Read the model definition and answer for the solid it produces. Units are mm, in the model's axes. Coordinates: 2 decimals unless noted, no trailing zeros. Write each loop counter-clockwise with the first axis right and the second up, starting at its lowest first coordinate (ties: lowest second). Pieces come first, ordered by that corner, then holes. Notation, with made-up numbers: (43.25, -24) -> (72.25, -24) arc R18 ccw to (72.25, -12) -> close; hole circle Ø10 at (-21.5, -27.75). An arc over 180 degrees is marked (long way). Write item = value, one per line. Start each with the question number.
1) Section B-B (x = 51) is taken. Determine the outline of the cut face in (y, z) (3 decimals).
2) For a pull along Y with two mould halves and no side action, classify faces 1 (the face through (6, -34, 0)), 2 (the face through (-6, -32.3, 0.5)) as released by +Y, released by -Y, zero draft, split by the parting line, or undercut.
3) Section C-C (z = 0.75) is taken. Determine the outline of the cut face in (x, y).
4) Section A-A (y = -4.5) is taken. Determine the outline of the cut face in (x, z).
5) A flat-ended cylindrical pin translates along its axis: pin 1 Ø6 at (x, y) = (-39, 26.5) entering from +Z. Find the tip coordinate at first contact, or state that the pin passes through.
6) Find the intervals of material crossed by line 1 along X through (y, z) = (7, 0.35); line 2 along Y through (x, z) = (65.5, 0.2) (3 decimals); line 3 along X through (y, z) = (-11, 0.9), in increasing order. Write a range as from..to.
from build123d import *

# Parameters (mm, degrees)
F0_W     = 152
F0_H     = 73
F1_DEPTH = 1
F0_W_2   = 150
F0_H_2   = 64.29
F2_DEPTH = 0.5


with BuildPart() as f1:
    # F0 (on Top) → F1 (new body)
    with BuildSketch(Plane.XY):
        Polygon((-78, -30), (-78, -38), (78, -38), (78, -30), (81, -30), (81, 38), (-81, 38), (-81, -30), align=None)
        Rectangle(F0_W, F0_H, mode=Mode.SUBTRACT)
    extrude(amount=F1_DEPTH)

    # F0 (on Top) → F2 (join)
    with BuildSketch(Plane.XY):
        Rectangle(F0_W, F0_H)
        Rectangle(F0_W_2, F0_H_2, mode=Mode.SUBTRACT)
    extrude(amount=F2_DEPTH)


solid = f1.part
Answer key:
q1.outline = (-38, 0) -> (-32.145, 0) -> (-32.145, 0.5) -> (-36.5, 0.5) -> (-36.5, 1) -> (-38, 1) -> close; (32.145, 0) -> (38, 0) -> (38, 1) -> (36.5, 1) -> (36.5, 0.5) -> (32.145, 0.5) -> close
q2.face_1 = zero draft
q2.face_2 = undercut
q3.outline = (-81, -30) -> (-78, -30) -> (-78, -38) -> (78, -38) -> (78, -30) -> (81, -30) -> (81, 38) -> (-81, 38) -> close; hole (-76, -36.5) -> (76, -36.5) -> (76, 36.5) -> (-76, 36.5) -> close
q4.outline = (-81, 0) -> (-75, 0) -> (-75, 0.5) -> (-76, 0.5) -> (-76, 1) -> (-81, 1) -> close; (75, 0) -> (81, 0) -> (81, 1) -> (76, 1) -> (76, 0.5) -> (75, 0.5) -> close
q5.pin_1 = through
q6.line_1 = -81..-75, 75..81
q6.line_2 = -38..-32.145, 32.145..38
q6.line_3 = -81..-76, 76..81
